Geometry: final body of the model. Coordinates: model frame, mm. Round coordinates to 2 decimals unless told otherwise and drop trailing zeros. Write each loop counter-clockwise with the first axis right and the second up, starting at its lowest first coordinate (ties: lowest second). Pieces come first, ordered by that corner, then holes. Notation, with made-up numbers: M 37.25,86.25 L 71.25,86.25 A17 cw 71.25,104.25 Z; hole C 17.5,24 d1. An arc over 180 degrees is marked long. Use one line per item in the form item = value. Start each with the question number.
from build123d import *

# Parameters (mm, degrees)
SKETCH1_W           = 240
SKETCH1_H           = 40
SKETCH1_R           = 2.05
SKETCH1_R_2         = 4
BOSS_EXTRUDE1_DEPTH = 3.175
FILLET1_R           = 2


with BuildPart() as part:
    # Sketch1 → Boss-Extrude1 (new body)
    with BuildSketch(Plane(origin=(0, 0, 0), x_dir=(1, 0, 0), z_dir=(0, 1, 0))):
        Rectangle(SKETCH1_W, SKETCH1_H)
        with Locations(Location((114.5, 16, 0), (0, 0, 270))):
            Circle(SKETCH1_R, mode=Mode.SUBTRACT)
        with Locations(Location((114.5, -16, 0), (0, 0, 270))):
            Circle(SKETCH1_R, mode=Mode.SUBTRACT)
        with Locations(Location((-114.5, 16, 0), (0, 0, 270))):
            Circle(SKETCH1_R, mode=Mode.SUBTRACT)
        with Locations(Location((-114.5, -16, 0), (0, 0, 270))):
            Circle(SKETCH1_R, mode=Mode.SUBTRACT)
        with Locations(Location((-52, -8, 0), (0, 0, 270))):
            Circle(SKETCH1_R, mode=Mode.SUBTRACT)
        with Locations(Location((-68, -8, 0), (0, 0, 270))):
            Circle(SKETCH1_R, mode=Mode.SUBTRACT)
        with Locations(Location((-68, 8, 0), (0, 0, 270))):
            Circle(SKETCH1_R, mode=Mode.SUBTRACT)
        with Locations(Location((-52, 8, 0), (0, 0, 270))):
            Circle(SKETCH1_R, mode=Mode.SUBTRACT)
        with Locations(Location((-60, 0, 0), (0, 0, 270))):
            Circle(SKETCH1_R_2, mode=Mode.SUBTRACT)
        with Locations(Location((68, 8, 0), (0, 0, 90))):
            Circle(SKETCH1_R, mode=Mode.SUBTRACT)
        with Locations(Location((52, 8, 0), (0, 0, 90))):
            Circle(SKETCH1_R, mode=Mode.SUBTRACT)
        with Locations(Location((60, 0, 0), (0, 0, 90))):
            Circle(SKETCH1_R_2, mode=Mode.SUBTRACT)
        with Locations(Location((68, -8, 0), (0, 0, 90))):
            Circle(SKETCH1_R, mode=Mode.SUBTRACT)
        with Locations(Location((52, -8, 0), (0, 0, 90))):
            Circle(SKETCH1_R, mode=Mode.SUBTRACT)
    extrude(amount=BOSS_EXTRUDE1_DEPTH)

    # Fillet1
    fillet1_edges = [part.edges().sort_by_distance(p)[0] for p in [
        (120, 1.5875, 20),
        (-120, 1.5875, 20),
        (-120, 1.5875, -20),
        (120, 1.5875, -20),
    ]]
    fillet(fillet1_edges, radius=FILLET1_R)


solid = part.part
1. Section query C-C (y = 2.15). Give the number of separate pieces and of enclosed holes in the cut face, then the cut area to 3 significant figures.
2. Section query A-A (z = 8). Return loops of the section in (x, y) (3 decimals), then the cut area to 3 significant figures.
3. Pull-direction query (X, two-part tool) for faces 1 (the face through (116.533, 1.565, -16.267)), 2 (the face through (-2, 3.175, 0)); classes: released by +X, released by -X, zero draft, split by the parting line, or undercut.
4. Section query D-D (z = -16). Return loops of the section in (x, y) (3 decimals), then the cut area to 3 significant figures.
5. Ray query, probe 1 along X at (y, z) = (1.3, -8); probe 2 along X at (y, z) = (0.4, 0); probe 3 along X at (y, z) = (1.65, 16). Return the intervals inside material, ascending.
6. Section query B-B (x = -60). Return loops of the section in (y, z) (3 decimals).
Checks:
q1.separate_pieces = 1
q1.enclosed_holes = 14
q1.area = 9,340 mm^2
q2.outline = M -120,0 L -70.05,0 L -70.05,3.175 L -120,3.175 Z; M -65.95,0 L -54.05,0 L -54.05,3.175 L -65.95,3.175 Z; M -49.95,0 L 49.95,0 L 49.95,3.175 L -49.95,3.175 Z; M 54.05,0 L 65.95,0 L 65.95,3.175 L 54.05,3.175 Z; M 70.05,0 L 120,0 L 120,3.175 L 70.05,3.175 Z
q2.area = 710 mm^2
q3.face_1 = undercut
q3.face_2 = zero draft
q4.outline = M -120,0 L -116.55,0 L -116.55,3.175 L -120,3.175 Z; M -112.45,0 L 112.45,0 L 112.45,3.175 L -112.45,3.175 Z; M 116.55,0 L 120,0 L 120,3.175 L 116.55,3.175 Z
q4.area = 736 mm^2
q5.probe_1 = -120 to -70.05, -65.95 to -54.05, -49.95 to 49.95, 54.05 to 65.95, 70.05 to 120
q5.probe_2 = -120 to -64, -56 to 56, 64 to 120
q5.probe_3 = -120 to -116.55, -112.45 to 112.45, 116.55 to 120
q6.outline = M 0,-20 L 3.175,-20 L 3.175,-4 L 0,-4 Z; M 0,4 L 3.175,4 L 3.175,20 L 0,20 Z
